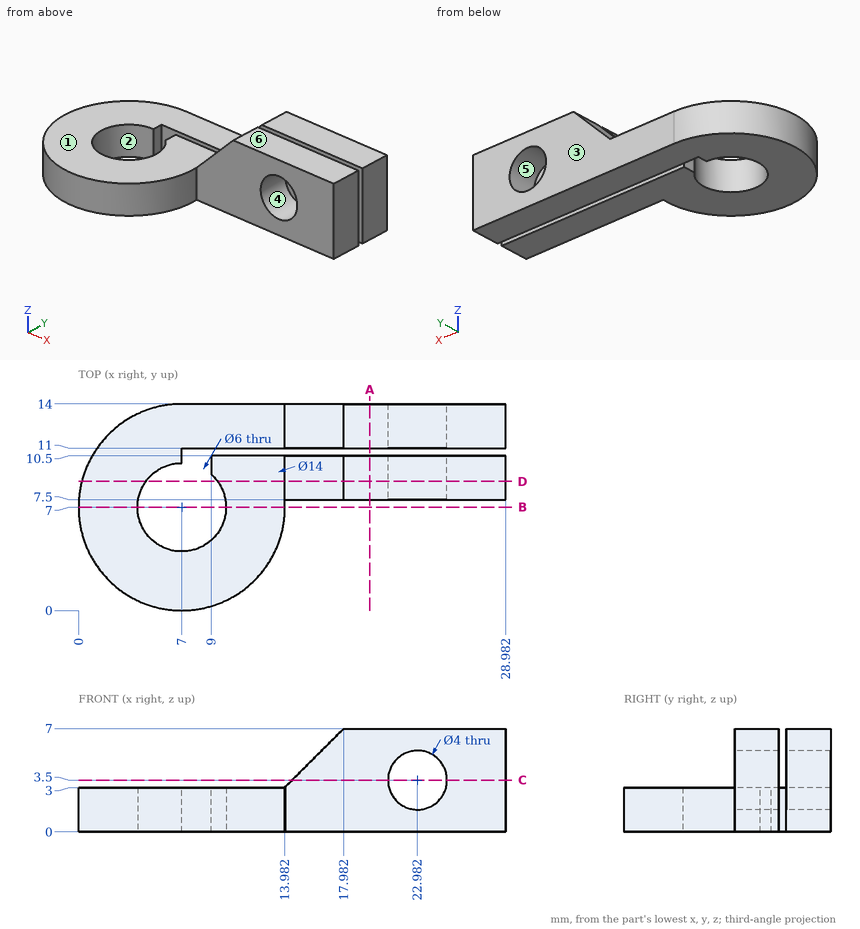
Drawing for the job (mm, zero at the part's lowest x, y, z). A direction names the side the tool comes from. Give positions to 0.01 mm unless a question says otherwise; leave off trailing zeros. Loops run counter-clockwise (first coordinate to the right, second up) from the corner with the lowest first, then second, coordinate; pieces in that order, holes last.
(1) Pin check, flat tips, straight feed: pin 1 (3 mm diameter, centred on y = 3.5, z = 2.5, fed in from -X); pin 2 (1.5 mm diameter, centred on y = 3, z = 1.5, fed in from +X); pin 3 (2 mm diameter, centred on x = 14.5, y = 7.5, fed in from +Z). Stop position of each tip, or through.
Return value:
pin 1: stops at x = 0.29
pin 2: stops at x = 13.2
pin 3: stops at z = 4.52
(2) Pull direction Z, two halves, no side cores. Call the marked faces 3, 4, 5 and 6: pulls with the +Z half, pulls with the -Z half, needs draft (parallel to the pull), parting line crosses it, or undercut.
Return value:
face 3: needs draft
face 4: undercut
face 5: undercut
face 6: pulls with the +Z half
(3) Band-saw the part on C-C (z = 3.5). Write the cut outline in (x, y).
Return value:
outline: (14.48, 7.5) - (20.98, 7.5) - (20.98, 10.5) - (14.48, 10.5) - close; (14.48, 11) - (20.98, 11) - (20.98, 14) - (14.48, 14) - close; (24.98, 7.5) - (28.98, 7.5) - (28.98, 10.5) - (24.98, 10.5) - close; (24.98, 11) - (28.98, 11) - (28.98, 14) - (24.98, 14) - close
(4) Band-saw the part on B-B (y = 7). Write the cut outline in (x, z).
Return value:
outline: (0, 0) - (4, 0) - (4, 3) - (0, 3) - close; (10, 0) - (14, 0) - (14, 3) - (10, 3) - close
(5) 3-axis set-ups, long thin cutter, end or side, ignore diameter. For the marked faces 1 and 2: which of +Z, -Z, +X, -X, +Y, -Y reach the whole face in a straight line?
Return value:
face 1: +Z, -X, +Y, -Y
face 2: +Z, -Z
(6) Band-saw the part on D-D (y = 8.75). Write the cut outline in (x, z), and give its area (3 significant figures).
Return value:
outline: (0.22, 0) - (4.56, 0) - (4.56, 3) - (0.22, 3) - close; (9.44, 0) - (28.98, 0) - (28.98, 7) - (17.98, 7) - (13.98, 3) - (9.44, 3) - close; hole circle Ø4 at (22.98, 3.5)
area: 111 mm2
(7) Band-saw the part on A-A (x = 19.75). Write the cut outline in (y, z), and give its area (3 significant figures).
Return value:
outline: (7.5, 0) - (10.5, 0) - (10.5, 7) - (7.5, 7) - close; (11, 0) - (14, 0) - (14, 7) - (11, 7) - close
area: 42.0 mm2
(8) Drill centre lines: line 1 along X through (y, z) = (7, 1.15); line 2 along Y through (x, z) = (20.5, 3.25); line 3 along Z through (x, y) = (21.75, 10.25) (1 decimal). Where is each one in solid material? Low to high.
Return value:
line 1: x = 0 to 4, 10 to 14
line 2: y = 7.5 to 10.5, 11 to 14
line 3: z = 0 to 1.9, 5.1 to 7
